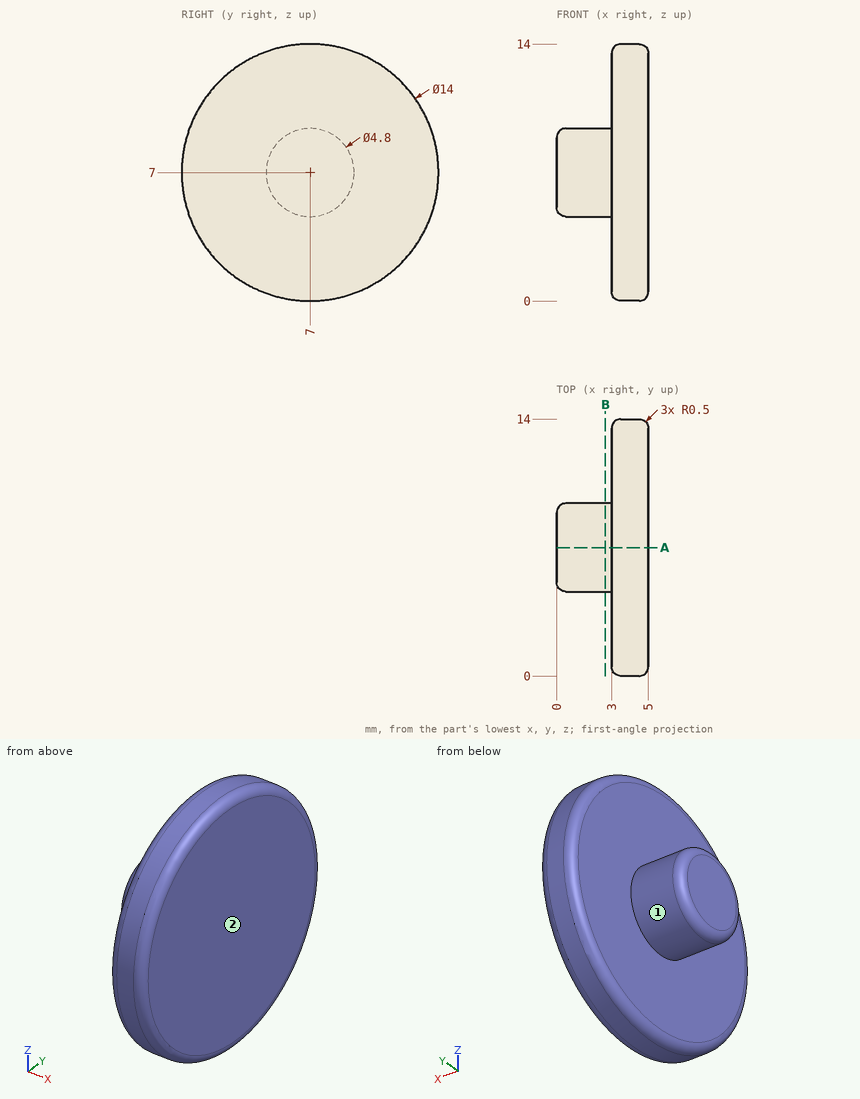
Could you check a few things on this drawing? It's one solid part, dimensions in mm from its lowest x, y, z. A direction names the side the tool comes from. Give positions to 0.01 mm unless a question says otherwise; leave off trailing zeros. Write each loop counter-clockwise with the first axis right and the second up, starting at its lowest first coordinate (ties: lowest second). Pieces come first, ordered by that corner, then holes. Notation, with made-up numbers: M -11.75,72 L 13.25,72 A25 ccw 13.25,94 Z; hole C -38.75,24 d11. An arc over 180 degrees is marked long. Put each result on its own line as item: value. Start each with the question number.
Item 1: If we section it at A-A, the plane y = 7: Write out the boundary of the cut face in (x, z).
Item 2: If we section it at B-B, the plane x = 2.65: Write out the boundary of the cut face in (y, z).
Item 3: I need wall thicknesses on L1, parallel to X at y = 5, z = 3.5; L2, parallel to Y at x = 2.2, z = 8.5; L3, parallel to Y at x = 4.6, z = 1.5. Which ranges of each line are inside material? Lowest first, please. Write a range as from..to.
Item 4: Will these pins go through, and if not, where does the flat tip stop? pin 1 (1.5 mm diameter, centred on x = 1, y = 9.5, fed in from -Z); pin 2 (2 mm diameter, centred on x = 4, z = 9.5, fed in from -Y); pin 3 (1.5 mm diameter, centred on x = 2, z = 8, fed in from +Y).
Item 5: On a 3-axis mill with a long thin cutter (end or side, diameter ignored), from which of +Z, -Z, +X, -X, +Y, -Y can I reach the whole of each face in a straight line? I mean the marked faces 1 and 2. Say none if no direction works.
Values:
1. outline: M 0,5.1 A0.5 ccw 0.5,4.6 L 3,4.6 L 3,0.5 A0.5 ccw 3.5,0 L 4.5,0 A0.5 ccw 5,0.5 L 5,13.5 A0.5 ccw 4.5,14 L 3.5,14 A0.5 ccw 3,13.5 L 3,9.4 L 0.5,9.4 A0.5 ccw 0,8.9 Z
2. outline: C 7,7 d4.8
3. L1: 3..5
3. L2: 5.13..8.87
3. L3: 2.69..11.31
4. pin 1: z = 5.36
4. pin 2: y = 0.16
4. pin 3: y = 9.39
5. face 1: -X
5. face 2: +Z, -Z, +X, +Y, -Y
